```python
from build123d import *

# Parameters (mm, degrees)
SKETCH1_R                 = 6
SKETCH1_R_2               = 3
BOSS_EXTRUDE1_DEPTH       = 4.2
SKETCH2_R                 = 12.7
SKETCH2_R_2               = 3
BOSS_EXTRUDE2_DEPTH       = 5
SKETCH3_R                 = 1.4
CUT_EXTRUDE1_DEPTH        = 13.7
F_4_40_TAPPED_HOLE1_D     = 2.2606
F_4_40_TAPPED_HOLE1_DEPTH = 7.6
F_4_40_TAPPED_HOLE1_TIP   = 0.679152758


with BuildPart() as part:
    # Sketch1 → Boss-Extrude1 (new body)
    with BuildSketch(Plane.XY):
        Circle(SKETCH1_R)
        Circle(SKETCH1_R_2, mode=Mode.SUBTRACT)
    extrude(amount=BOSS_EXTRUDE1_DEPTH)

    # Sketch2 → Boss-Extrude2 (add)
    with BuildSketch(Plane.XY.offset(4.2)):
        Circle(SKETCH2_R)
        Circle(SKETCH2_R_2, mode=Mode.SUBTRACT)
    extrude(amount=BOSS_EXTRUDE2_DEPTH)

    # Sketch3 → Cut-Extrude1 (cut, through all)
    with BuildSketch(Plane(origin=(0, 0, 0), x_dir=(1, 0, 0), z_dir=(0, 1, 0))):
        with Locations((0, -2.1)):
            Circle(SKETCH3_R)
    extrude(amount=-CUT_EXTRUDE1_DEPTH, mode=Mode.SUBTRACT)

    # #4-40 Tapped Hole1
    with Locations(Plane.XY.offset(9.2)):
        with Locations((-8.227241336, -4.75), (-8.227241336, 4.75), (0, 9.5), (8.227241336, 4.75), (8.227241336, -4.75), (0, -9.5)):
            Hole(F_4_40_TAPPED_HOLE1_D / 2, depth=F_4_40_TAPPED_HOLE1_DEPTH)
            with Locations((0, 0, -(F_4_40_TAPPED_HOLE1_DEPTH + F_4_40_TAPPED_HOLE1_TIP / 2))):  # 118° drill point
                Cone(0, F_4_40_TAPPED_HOLE1_D / 2, F_4_40_TAPPED_HOLE1_TIP, mode=Mode.SUBTRACT)


solid = part.part
```
Check sheet for the modelled part. Datum: model origin and axes. Units: mm. A direction names the side the tool comes from. Round coordinates to 2 decimals unless told otherwise and drop trailing zeros. Loops run counter-clockwise (first coordinate to the right, second up) from the corner with the lowest first, then second, coordinate; pieces in that order, holes last. Notation, with made-up numbers: (-14, 36) -> (27, 36) arc R33 cw to (27, 67) -> close; hole circle Ø6 at (64, -38). An arc over 180 degrees is marked (long way). Answer in a Markdown table with one row per item.
Q1. Release check for a two-part mould opening along X. For faces 4 (the face through (7.18, -5.18, 6.66)), 5 (the face through (-2.75, -12.4, 6.66)), 6 (the face through (-3, -5.5, 4.2)) record: released by +X, released by -X, zero draft, split by the parting line, or undercut.
Data:
| item | result |
|---|---|
| face 4 | undercut |
| face 5 | split by the parting line |
| face 6 | zero draft |
Q2. Sectioned sample at D-D on y = 4.75. Enter the section's corners in (x, z), then the cut area to 3 significant figures.
Data:
| item | result |
|---|---|
| outline | (-11.78, 4.2) -> (-9.36, 4.2) -> (-9.36, 9.2) -> (-11.78, 9.2) -> close; (-7.1, 4.2) -> (-3.67, 4.2) -> (-3.67, 0) -> (3.67, 0) -> (3.67, 4.2) -> (7.1, 4.2) -> (7.1, 9.2) -> (-7.1, 9.2) -> close; (9.36, 4.2) -> (11.78, 4.2) -> (11.78, 9.2) -> (9.36, 9.2) -> close |
| area | 126 mm^2 |
Q3. Sectioned sample at A-A on y = -4.75. Enter the section's corners in (x, z).
Data:
| item | result |
|---|---|
| outline | (-11.78, 4.2) -> (-9.36, 4.2) -> (-9.36, 9.2) -> (-11.78, 9.2) -> close; (-7.1, 4.2) -> (-3.67, 4.2) -> (-3.67, 0) -> (3.67, 0) -> (3.67, 4.2) -> (7.1, 4.2) -> (7.1, 9.2) -> (-7.1, 9.2) -> close; (9.36, 4.2) -> (11.78, 4.2) -> (11.78, 9.2) -> (9.36, 9.2) -> close; hole circle Ø2.8 at (0, 2.1) |
Q4. Set-up check for faces 1 (the face through (-0.78, 5.95, 2.07)), 2 (the face through (0, 3, 5)), 3 (the face through (-0.303, -4.305, 3.467)): record each of +Z, -Z, +X, -X, +Y, -Y from which the full face is reachable in a straight line by a thin tool's end or side.
Data:
| item | result |
|---|---|
| face 1 | -Z |
| face 2 | +Z, -Z |
| face 3 | -Y |
Q5. Thickness scan on L1, parallel to Y at x = 0, z = 5.75; L2, parallel to Y at x = 8.5, z = 5.25; L3, parallel to X at y = 5, z = 6. Record the ranges inside material, lowest first.
Data:
| item | result |
|---|---|
| L1 | y = -12.7 to -10.63, -8.37 to -3, 3 to 8.37, 10.63 to 12.7 |
| L2 | y = -9.44 to -5.85, -3.65 to 3.65, 5.85 to 9.44 |
| L3 | x = -11.67 to -9.33, -7.12 to 7.12, 9.33 to 11.67 |
Q6. Go/stop test with flat-tipped pins: P1, Ø1.8, axis at x = 0, y = -9.5, coming from the -Z side; P2, Ø3.5, axis at x = 8.23, y = 4.75, coming from the -Z side; P3, Ø5, axis at y = -4.5, z = 2, coming from the -X side; P4, Ø2, axis at x = 6.5, z = 6, coming from the -Y side. Record where each tip stops, or that it passes through.
Data:
| item | result |
|---|---|
| P1 | passes through |
| P2 | stops at z = 4.2 |
| P3 | stops at x = -12.26 |
| P4 | stops at y = -11.45 |
Q7. Sectioned sample at C-C on y = 0. Enter the section's corners in (x, z).
Data:
| item | result |
|---|---|
| outline | (-12.7, 4.2) -> (-6, 4.2) -> (-6, 0) -> (-3, 0) -> (-3, 9.2) -> (-12.7, 9.2) -> close; (3, 0) -> (6, 0) -> (6, 4.2) -> (12.7, 4.2) -> (12.7, 9.2) -> (3, 9.2) -> close |
Q8. Sectioned sample at B-B on z = 5.5. Enter the section's corners in (x, y), then the cut area to 3 significant figures.
Data:
| item | result |
|---|---|
| outline | circle Ø25.4 at (0, 0); hole circle Ø2.26 at (-8.23, -4.75); hole circle Ø2.26 at (-8.23, 4.75); hole circle Ø6 at (0, 0); hole circle Ø2.26 at (0, -9.5); hole circle Ø2.26 at (0, 9.5); hole circle Ø2.26 at (8.23, -4.75); hole circle Ø2.26 at (8.23, 4.75) |
| area | 454 mm^2 |
